For this review, take the finished solid that the model builds, in its own axes (mm). A direction names the side the tool comes from. Round coordinates to 2 decimals unless told otherwise and drop trailing zeros. Loops run counter-clockwise (first coordinate to the right, second up) from the corner with the lowest first, then second, coordinate; pieces in that order, holes last. Notation, with made-up numbers: (-23, 60) -> (16, 60) arc R17 cw to (16, 70) -> close; hole circle Ø2 at (-20.5, 37). An arc over 180 degrees is marked (long way). One line per question, with ' | ' between items. Start each with the question number.
1. For pin 1 Ø4 at (x, y) = (7.5, -12.99) entering from -Z; pin 2 Ø12 at (y, z) = (7.5, -7.5) entering from -X; pin 3 Ø5 at (x, z) = (13, -14.5) entering from -Y, all flat-tipped, find the tip position at first contact; note any pin that passes through.
2. Wall thickness on line 1 along Y through (x, z) = (-7.5, -2.25); line 2 along Y through (x, z) = (-7, -5); line 3 along Z through (x, y) = (-2.5, 7): over which ranges is each line inside the solid? List them lowest first.
3. Consider section A-A (z = -5). Write out the cut boundary in (x, y).
4. Consider section B-B (z = -32). Write out the cut boundary in (x, y), and give its area (3 significant figures).
5. Draft analysis for pull direction Y (two halves, no side actions). For faces 1 (the face through (-8, 13, -10)), 2 (the face through (1, 10, 6)), 3 (the face through (1.08, -4.88, -52.71)), state which applies: pulls with the +Y half, pulls with the -Y half, needs draft (parallel to the pull), parting line crosses it, or undercut.
6. For faces 4 (the face through (-8.61, 14, -4.93)), 5 (the face through (-4.01, -18.06, -14.8)), list the 3-axis set-ups (+Z, -Z, +X, -X, +Y, -Y) from which the entire face can be reached by the end or side of a thin tool; tool diameter is ignored.
```python
from build123d import *

# Parameters (mm, degrees)
SKETCH_1_R          = 18.5
EXTRUDE_1_DEPTH     = 50
SKETCH_2_R          = 5
EXTRUDE_2_DEPTH     = 6
EXTRUDE_3_DEPTH     = 21
CUT_EXTRUDE_1_DEPTH = 10
SKETCH_5_R          = 6
EXTRUDE_4_DEPTH     = 6
CUT_EXTRUDE_START   = -30
CUT_EXTRUDE_2_DEPTH = 20
SKETCH_8_R          = 1.5
CUT_EXTRUDE_3_DEPTH = 10


with BuildPart() as part:
    # 草图1 → 凸台-拉伸1 (new body)
    with BuildSketch(Plane.XY):
        Circle(SKETCH_1_R)
    extrude(amount=-EXTRUDE_1_DEPTH)

    # 草图2 → 凸台-拉伸2 (add)
    with BuildSketch(Plane(origin=(0, 0, -50), x_dir=(-1, 0, 0), z_dir=(0, 0, -1))):
        Circle(SKETCH_2_R)
    extrude(amount=EXTRUDE_2_DEPTH)

    # 草图1<3> → 凸台-拉伸3 (add)
    with BuildSketch(Plane.XY):
        with BuildLine():
            ThreePointArc((0, 10), (-3, 7), (0, 4))
            Line((0, 4), (0, 10))
        make_face()
        with BuildLine():
            Line((0, 10), (0, 4))
            ThreePointArc((0, 4), (2.121320344, 4.878679656), (3, 7))
            ThreePointArc((3, 7), (2.121320344, 9.121320344), (0, 10))
        make_face()
    extrude(amount=EXTRUDE_3_DEPTH)

    # 草图4 → 切除-拉伸1 (cut)
    with BuildSketch(Plane.XY.offset(21)):
        Polygon((-80.661429966, 9.5), (-1.658312395, 9.5), (1.658312395, 9.5), (80.661429966, 9.5), (80.661429966, 167.506235142), (-80.661429966, 167.506235142), align=None)
    extrude(amount=-CUT_EXTRUDE_1_DEPTH, mode=Mode.SUBTRACT)

    # 草图5 → 凸台-拉伸4 (add)
    with BuildSketch(Plane.XY):
        with Locations((0, 7)):
            Circle(SKETCH_5_R)
    extrude(amount=EXTRUDE_4_DEPTH)

    # 草图1<5> → 切除-拉伸2 (cut)
    with BuildSketch(Plane.XY.offset(CUT_EXTRUDE_START)):
        with BuildLine():
            ThreePointArc((0, 18.5), (-18.5, 0), (0, -18.5))
            Line((0, -18.5), (0, -17.5))
            ThreePointArc((0, -17.5), (-17.5, 0), (0, 17.5))
            Line((0, 17.5), (0, 18.5))
        make_face()
        with BuildLine():
            Line((0, -17.5), (0, -18.5))
            ThreePointArc((0, -18.5), (13.081475452, -13.081475452), (18.5, 0))
            ThreePointArc((18.5, 0), (13.081475452, 13.081475452), (0, 18.5))
            Line((0, 18.5), (0, 17.5))
            ThreePointArc((0, 17.5), (12.374368671, 12.374368671), (17.5, 0))
            ThreePointArc((17.5, 0), (12.374368671, -12.374368671), (0, -17.5))
        make_face()
    extrude(amount=-CUT_EXTRUDE_2_DEPTH, mode=Mode.SUBTRACT)

    # 倒角1: read off the stored shape, not the designer's step
    # 倒角1 outline → 倒角1 (revolve, cut)
    with BuildSketch(Plane.XZ):
        Polygon((5, -55.5), (4.5, -56), (5, -56), align=None)
        Polygon((17.5, -49.5), (17, -50), (17.5, -50), align=None)
        Polygon((18.5, -29.5), (18, -30), (18.5, -30), align=None)
        Polygon((18, 0), (18.5, -0.5), (18.5, 0), align=None)
    revolve(axis=Axis((0, 0, 0), (0, 0, 1)), mode=Mode.SUBTRACT)

    # 草图8 → 切除-拉伸3 (cut)
    with BuildSketch(Plane.XY):
        with Locations((15, 0)):
            Circle(SKETCH_8_R)
        with Locations((7.5, -12.990381057)):
            Circle(SKETCH_8_R)
        with Locations((-7.5, -12.990381057)):
            Circle(SKETCH_8_R)
        with Locations((-15, 0)):
            Circle(SKETCH_8_R)
        with Locations((-7.5, 12.990381057)):
            Circle(SKETCH_8_R)
        with Locations((7.5, 12.990381057)):
            Circle(SKETCH_8_R)
    extrude(amount=-CUT_EXTRUDE_3_DEPTH, mode=Mode.SUBTRACT)


solid = part.part
```
Answer block:
1) pin 1: stops at z = -50 | pin 2: stops at x = -18.44 | pin 3: stops at y = -15.23
2) line 1: y = -16.91 to -14.49, -11.49 to 11.49, 14.49 to 16.91 | line 2: y = -17.12 to -14.4, -11.58 to 11.58, 14.4 to 17.12 | line 3: z = -50 to 21
3) outline: circle Ø37 at (0, 0); hole circle Ø3 at (-15, 0); hole circle Ø3 at (-7.5, -12.99); hole circle Ø3 at (-7.5, 12.99); hole circle Ø3 at (7.5, -12.99); hole circle Ø3 at (7.5, 12.99); hole circle Ø3 at (15, 0)
4) outline: circle Ø35 at (0, 0) | area: 962 mm2
5) face 1: undercut | face 2: needs draft | face 3: parting line crosses it
6) face 4: +Z | face 5: +Z, -Z
